Read the model definition and answer for the solid it produces. Units are mm, in the model's axes. Coordinates: 2 decimals unless noted, no trailing zeros. Loops run counter-clockwise (first coordinate to the right, second up) from the corner with the lowest first, then second, coordinate; pieces in that order, holes last.
from build123d import *

# Parameters (mm, degrees)
F0_W     = 100
F0_H     = 175
F0_R     = 2.55
F1_DEPTH = 6
F2_R     = 5


with BuildPart() as f1:
    # F0 (on Front) → F1 (new body)
    with BuildSketch(Plane.XZ):
        Rectangle(F0_W, F0_H)
        with Locations((-43, -80.5)):
            Circle(F0_R, mode=Mode.SUBTRACT)
        with Locations((43, -80.5)):
            Circle(F0_R, mode=Mode.SUBTRACT)
        with Locations((-43, 80.5)):
            Circle(F0_R, mode=Mode.SUBTRACT)
        with Locations((43, 80.5)):
            Circle(F0_R, mode=Mode.SUBTRACT)
    extrude(amount=F1_DEPTH)

    # F2
    f2_edges = [f1.edges().sort_by_distance(p)[0] for p in [
        (-50, -3, 87.5),
        (-50, -3, -87.5),
        (50, -3, 87.5),
        (50, -3, -87.5),
    ]]
    fillet(f2_edges, radius=F2_R)


solid = f1.part
Item 1: Given pin 1 (3 mm diameter, centred on x = 43, z = -80.5, fed in from +Y), flat-ended and moving along its own axis, determine where the tip first touches the part or whether it passes through.
Numbers:
pin 1: passes through
Item 2: A cutting plane is placed at A-A on x = -43. Determine the outline of the cut face in (y, z).
Numbers:
outline: (-6, -87.5) - (0, -87.5) - (0, -83.05) - (-6, -83.05) - close; (-6, -77.95) - (0, -77.95) - (0, 77.95) - (-6, 77.95) - close; (-6, 83.05) - (0, 83.05) - (0, 87.5) - (-6, 87.5) - close
Item 3: Determine the mould class of faces 1 (the face through (-45.548, -2.958, -80.388)), 2 (the face through (-1, 0, 1)), 3 (the face through (40.452, -2.958, -80.388)), 4 (the face through (-48.57, -3.04, -86)) for opening direction Z: released by +Z, released by -Z, zero draft, split by the parting line, or undercut.
Numbers:
face 1: undercut
face 2: zero draft
face 3: undercut
face 4: released by -Z
Item 4: Find the intervals of material crossed by line 1 along Z through (x, y) = (-43, -1.15), in increasing order.
Numbers:
line 1: z = -87.5 to -83.05, -77.95 to 77.95, 83.05 to 87.5
Item 5: A cutting plane is placed at B-B on z = 80.5. Determine the outline of the cut face in (x, y), then the cut area to 3 significant figures.
Numbers:
outline: (-50, -6) - (-45.55, -6) - (-45.55, 0) - (-50, 0) - close; (-40.45, -6) - (40.45, -6) - (40.45, 0) - (-40.45, 0) - close; (45.55, -6) - (50, -6) - (50, 0) - (45.55, 0) - close
area: 539 mm2
